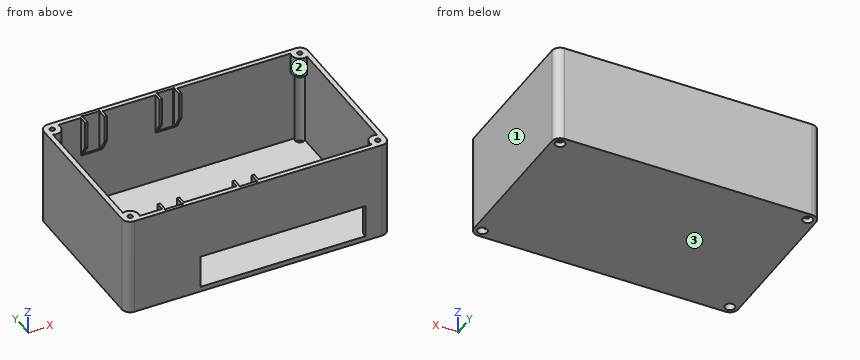
from build123d import *
from OCP.BRepFilletAPI import BRepFilletAPI_MakeChamfer

# Parameters (mm, degrees)
BASESHAPE_W                = 160
BASESHAPE_H                = 100
CONTAINERBASE_DEPTH        = 60
SIDECORNERFILLET_R         = 5
CONTAINERSHELL_T           = -3
SLOTSKETCH_W               = 10.2
SLOTSKETCH_H               = 25
SLOTCUT_DEPTH              = 1
VIEWELECTRONICSHOLE_REACH  = 199.99
ELECTRONICSVIEWHOLE_W      = 100
ELECTRONICSVIEWHOLE_H      = 20
SCREWSUPPORTS_R            = 5
BOSS_EXTRUDE3_DEPTH        = 15
SCREWSUPPORTTAPER_SIZE     = 3
SKETCH5_R                  = 3
COUNTERSINKCUT_DEPTH       = 52
SKETCH6_R                  = 1.5
SCREWHOLES_DEPTH           = 52
SKETCH7_W                  = 1.5
SKETCH7_H                  = 25
BOSS_EXTRUDE4_DEPTH        = 5
CHAMFER1_SIZE              = 8.660254038
CHAMFER1_SIZE_2            = 5
CHAMFER1_OF_MIRROR3_SIZE   = 5
CHAMFER1_OF_MIRROR3_SIZE_2 = 8.660254038
SKETCH8_R                  = 0.375
CUT_EXTRUDE1_DEPTH         = 25


with BuildPart() as part:
    # BaseShape → ContainerBase (new body)
    with BuildSketch(Plane.XY):
        with Locations((-80, -50)):
            Rectangle(BASESHAPE_W, BASESHAPE_H)
    extrude(amount=CONTAINERBASE_DEPTH)

    # SideCornerFillet
    sidecornerfillet_edges = [part.edges().sort_by_distance(p)[0] for p in [
        (0, -100, 30),
        (-160, -100, 30),
        (-160, 0, 30),
        (0, 0, 30),
    ]]
    fillet(sidecornerfillet_edges, radius=SIDECORNERFILLET_R)

    # ContainerShell
    containershell_openings = [part.faces().sort_by_distance(p)[0] for p in [
        (-80, -50, 60),
    ]]
    offset(amount=CONTAINERSHELL_T, openings=containershell_openings, kind=Kind.INTERSECTION)

    # SlotSketch → SlotCut (cut)
    with BuildSketch(Plane.XZ.offset(3)):
        with Locations((-130.1, 47.5)):
            Rectangle(SLOTSKETCH_W, SLOTSKETCH_H)
        with Locations((-84.9, 47.5)):
            Rectangle(SLOTSKETCH_W, SLOTSKETCH_H)
    slotcut = extrude(amount=-SLOTCUT_DEPTH, mode=Mode.SUBTRACT)

    # MirrorSlots: SlotCut across plane
    add(slotcut.mirror(Plane(origin=(0, -50, 0), x_dir=(0, 0, 1), z_dir=(0, -1, 0))), mode=Mode.SUBTRACT)

    # ElectronicsViewHole → ViewElectronicsHole (cut, up to next)
    with BuildSketch(Plane.XZ.offset(100), mode=Mode.PRIVATE) as viewelectronicshole_sk1:
        with Locations((-65, 13)):
            Rectangle(ELECTRONICSVIEWHOLE_W, ELECTRONICSVIEWHOLE_H)
    viewelectronicshole_tool1 = extrude(viewelectronicshole_sk1.sketch, amount=-VIEWELECTRONICSHOLE_REACH, mode=Mode.PRIVATE) & part.part
    add(viewelectronicshole_tool1.solids().sort_by_distance((-65, -100, 13))[0], mode=Mode.SUBTRACT)

    # ScrewSupports → Boss-Extrude3 (add)
    with BuildSketch(Plane.XY.offset(60)):
        with Locations((-155, -5)):
            Circle(SCREWSUPPORTS_R)
        with Locations((-155, -95)):
            Circle(SCREWSUPPORTS_R)
        with Locations((-5, -95)):
            Circle(SCREWSUPPORTS_R)
        with Locations((-5, -5)):
            Circle(SCREWSUPPORTS_R)
    extrude(amount=-BOSS_EXTRUDE3_DEPTH)

    # ScrewSupportTaper
    screwsupporttaper_edges = [part.edges().sort_by_distance(p)[0] for p in [
        (-151.464466094, -8.535533906, 45),
        (-8.535533906, -91.464466094, 45),
        (-8.535533906, -8.535533906, 45),
        (-151.464466094, -91.464466094, 45),
    ]]
    chamfer(screwsupporttaper_edges, length=SCREWSUPPORTTAPER_SIZE)

    # Sketch5 → CounterSinkCut (cut)
    with BuildSketch(Plane(origin=(0, 0, 0), x_dir=(-1, 0, 0), z_dir=(0, 0, -1))):
        with Locations((5, -5)):
            Circle(SKETCH5_R)
        with Locations((5, -95)):
            Circle(SKETCH5_R)
        with Locations((155, -95)):
            Circle(SKETCH5_R)
        with Locations((155, -5)):
            Circle(SKETCH5_R)
    extrude(amount=-COUNTERSINKCUT_DEPTH, mode=Mode.SUBTRACT)

    # Sketch6 → ScrewHoles (cut)
    with BuildSketch(Plane.XY.offset(60)):
        with Locations((-155, -5)):
            Circle(SKETCH6_R)
        with Locations((-155, -95)):
            Circle(SKETCH6_R)
        with Locations((-5, -95)):
            Circle(SKETCH6_R)
        with Locations((-5, -5)):
            Circle(SKETCH6_R)
    extrude(amount=-SCREWHOLES_DEPTH, mode=Mode.SUBTRACT)

    # Sketch7 → Boss-Extrude4 (add)
    with BuildSketch(Plane.XZ.offset(3)):
        with Locations((-135.95, 47.5)):
            Rectangle(SKETCH7_W, SKETCH7_H)
        with Locations((-124.25, 47.5)):
            Rectangle(SKETCH7_W, SKETCH7_H)
        with Locations((-90.75, 47.5)):
            Rectangle(SKETCH7_W, SKETCH7_H)
        with Locations((-79.05, 47.5)):
            Rectangle(SKETCH7_W, SKETCH7_H)
    boss_extrude4 = extrude(amount=BOSS_EXTRUDE4_DEPTH)

    # Chamfer1
    chamfer1_edges_1 = [part.edges().sort_by_distance(p)[0] for p in [
        (-135.95, -8, 35),
    ]]
    chamfer1_side_1 = [part.faces().sort_by_distance(p)[0] for p in [
        (-135.95, -8, 35.1),
    ]]
    chamfer1_edges_2 = [part.edges().sort_by_distance(p)[0] for p in [
        (-124.25, -8, 35),
    ]]
    chamfer1_side_2 = [part.faces().sort_by_distance(p)[0] for p in [
        (-124.25, -8, 35.1),
    ]]
    chamfer1_edges_3 = [part.edges().sort_by_distance(p)[0] for p in [
        (-79.05, -8, 35),
    ]]
    chamfer1_side_3 = [part.faces().sort_by_distance(p)[0] for p in [
        (-79.05, -8, 35.1),
    ]]
    chamfer1_edges_4 = [part.edges().sort_by_distance(p)[0] for p in [
        (-90.75, -8, 35),
    ]]
    chamfer1_side_4 = [part.faces().sort_by_distance(p)[0] for p in [
        (-90.75, -8, 35.1),
    ]]
    chamfer1 = BRepFilletAPI_MakeChamfer(part.part.solid().wrapped)
    for e in chamfer1_edges_1:
        chamfer1.Add(CHAMFER1_SIZE - 0.0001, CHAMFER1_SIZE_2 - 0.0001, e.wrapped, chamfer1_side_1[0].wrapped)
    for e in chamfer1_edges_2:
        chamfer1.Add(CHAMFER1_SIZE - 0.0001, CHAMFER1_SIZE_2 - 0.0001, e.wrapped, chamfer1_side_2[0].wrapped)
    for e in chamfer1_edges_3:
        chamfer1.Add(CHAMFER1_SIZE - 0.0001, CHAMFER1_SIZE_2 - 0.0001, e.wrapped, chamfer1_side_3[0].wrapped)
    for e in chamfer1_edges_4:
        chamfer1.Add(CHAMFER1_SIZE - 0.0001, CHAMFER1_SIZE_2 - 0.0001, e.wrapped, chamfer1_side_4[0].wrapped)
    add(Compound.cast(chamfer1.Shape()), mode=Mode.REPLACE)  # a hair under: the kernel refuses the full size

    # Mirror3: Boss-Extrude4 across plane
    add(boss_extrude4.mirror(Plane.ZX.offset(-50)))

    # Chamfer1 of Mirror3
    chamfer1_of_mirror3_edges_1 = [part.edges().sort_by_distance(p)[0] for p in [
        (-135.95, -92, 35),
    ]]
    chamfer1_of_mirror3_side_1 = [part.faces().sort_by_distance(p)[0] for p in [
        (-135.95, -92.1, 35),
    ]]
    chamfer1_of_mirror3_edges_2 = [part.edges().sort_by_distance(p)[0] for p in [
        (-124.25, -92, 35),
    ]]
    chamfer1_of_mirror3_side_2 = [part.faces().sort_by_distance(p)[0] for p in [
        (-124.25, -92.1, 35),
    ]]
    chamfer1_of_mirror3_edges_3 = [part.edges().sort_by_distance(p)[0] for p in [
        (-79.05, -92, 35),
    ]]
    chamfer1_of_mirror3_side_3 = [part.faces().sort_by_distance(p)[0] for p in [
        (-79.05, -92.1, 35),
    ]]
    chamfer1_of_mirror3_edges_4 = [part.edges().sort_by_distance(p)[0] for p in [
        (-90.75, -92, 35),
    ]]
    chamfer1_of_mirror3_side_4 = [part.faces().sort_by_distance(p)[0] for p in [
        (-90.75, -92.1, 35),
    ]]
    chamfer1_of_mirror3 = BRepFilletAPI_MakeChamfer(part.part.solid().wrapped)
    for e in chamfer1_of_mirror3_edges_1:
        chamfer1_of_mirror3.Add(CHAMFER1_OF_MIRROR3_SIZE - 0.0001, CHAMFER1_OF_MIRROR3_SIZE_2 - 0.0001, e.wrapped, chamfer1_of_mirror3_side_1[0].wrapped)
    for e in chamfer1_of_mirror3_edges_2:
        chamfer1_of_mirror3.Add(CHAMFER1_OF_MIRROR3_SIZE - 0.0001, CHAMFER1_OF_MIRROR3_SIZE_2 - 0.0001, e.wrapped, chamfer1_of_mirror3_side_2[0].wrapped)
    for e in chamfer1_of_mirror3_edges_3:
        chamfer1_of_mirror3.Add(CHAMFER1_OF_MIRROR3_SIZE - 0.0001, CHAMFER1_OF_MIRROR3_SIZE_2 - 0.0001, e.wrapped, chamfer1_of_mirror3_side_3[0].wrapped)
    for e in chamfer1_of_mirror3_edges_4:
        chamfer1_of_mirror3.Add(CHAMFER1_OF_MIRROR3_SIZE - 0.0001, CHAMFER1_OF_MIRROR3_SIZE_2 - 0.0001, e.wrapped, chamfer1_of_mirror3_side_4[0].wrapped)
    add(Compound.cast(chamfer1_of_mirror3.Shape()), mode=Mode.REPLACE)  # a hair under: the kernel refuses the full size

    # Sketch8 → Cut-Extrude1 (cut)
    with BuildSketch(Plane.XY.offset(60)):
        with Locations((-135.2, -2)):
            Circle(SKETCH8_R)
        with Locations((-125, -2)):
            Circle(SKETCH8_R)
        with Locations((-90, -2)):
            Circle(SKETCH8_R)
        with Locations((-79.8, -2)):
            Circle(SKETCH8_R)
        with Locations((-135.2, -98)):
            Circle(SKETCH8_R)
        with Locations((-90, -98)):
            Circle(SKETCH8_R)
        with Locations((-125, -98)):
            Circle(SKETCH8_R)
        with Locations((-79.8, -98)):
            Circle(SKETCH8_R)
    extrude(amount=-CUT_EXTRUDE1_DEPTH, mode=Mode.SUBTRACT)


solid = part.part
Work out the finished part from the listing and answer in its coordinate system (mm). Face numbers are marked on the shaded views. Round coordinates to 2 decimals unless told otherwise and drop trailing zeros. Order: outer loops, then holes, each group sorted by start corner. A loop starts at its lowest first (then second) coordinate and runs counter-clockwise, first axis right, second up. Notation, with made-up numbers: M 42.25,34.25 L 73.25,34.25 A21 ccw 73.25,60.25 Z; hole C 54.25,11.5 d3. An arc over 180 degrees is marked long. Put each result on its own line as item: value. Start each with the question number.
Q1. Section B-B, the plane z = 16 is taken. Write down the section's boundary in (x, y), and give its area (3 significant figures).
Q2. Section A-A, the plane z = 32.5 is taken. Write down the section's boundary in (x, y), and give its area (3 significant figures).
Q3. For a pull along X with two mould halves and no side action, classify the marked faces 1, 2 and 3 as pulls with the +X half, pulls with the -X half, needs draft (parallel to the pull), parting line crosses it, or undercut.
Q4. Section C-C, the plane y = -28.5 is taken. Write down the section's boundary in (x, z), and give its area (3 significant figures).
Q5. Flat-ended cylindrical pins translate along their axes: pin 1 (4 mm diameter, centred on x = -31.5, y = -81.5, fed in from +Z); pin 2 (2.5 mm diameter, centred on x = -155, y = -5, fed in from -Z). Find the tip coordinate at first contact, or state that the pin passes through.
Q6. Straight lines are drawn through the part: L1, parallel to X at y = -62, z = 5; L2, parallel to Y at x = -143, z = 4.5; L3, parallel to Y at x = -113.5, z = 9. For each, find the intervals that lie inside material, in ascending order. Write a range as [from, to].
Findings below:
1. outline: M -160,-95 A5 ccw -155,-100 L -115,-100 L -115,-97 L -152.76,-97 A3 cw long -157,-92.76 L -157,-7.24 A3 cw long -152.76,-3 L -7.24,-3 A3 cw long -3,-7.24 L -3,-92.76 A3 cw long -7.24,-97 L -15,-97 L -15,-100 L -5,-100 A5 ccw 0,-95 L 0,-5 A5 ccw -5,0 L -155,0 A5 ccw -160,-5 Z
1. area: 1,180 mm^2
2. outline: M -160,-95 A5 ccw -155,-100 L -5,-100 A5 ccw 0,-95 L 0,-5 A5 ccw -5,0 L -155,0 A5 ccw -160,-5 Z; hole M -157,-92.76 A3 ccw long -152.76,-97 L -7.24,-97 A3 ccw long -3,-92.76 L -3,-7.24 A3 ccw long -7.24,-3 L -152.76,-3 A3 ccw long -157,-7.24 Z
2. area: 1,480 mm^2
3. face 1: pulls with the +X half
3. face 2: undercut
3. face 3: needs draft
4. outline: M -160,0 L 0,0 L 0,60 L -3,60 L -3,3 L -157,3 L -157,60 L -160,60 Z
4. area: 822 mm^2
5. pin 1: stops at z = 3
5. pin 2: passes through
6. L1: x = [-160, -157], [-3, 0]
6. L2: y = [-100, -97], [-3, 0]
6. L3: y = [-3, 0]
